```python
from build123d import *

# Parameters (mm, degrees)
CYLINDER005_R          = 1.7
CYLINDER005_DEPTH      = 20
CYLINDER004_R          = 1.7
CYLINDER004_DEPTH      = 36.75
CYLINDER003_R          = 1.7
CYLINDER003_DEPTH      = 39.75
CYLINDER006_R          = 1.7
CYLINDER006_DEPTH      = 20
CYLINDER001_R          = 8
CYLINDER001_DEPTH      = 5
CYLINDER001_ROLL_ANGLE = -90
CYLINDER_R             = 6
CYLINDER_DEPTH         = 30
CYLINDER_ROLL_ANGLE    = -90
CYLINDER002_R          = 8
CYLINDER002_DEPTH      = 12
CYLINDER002_ROLL_ANGLE = -90
BOX_W                  = 50
BOX_H                  = 15.9
BOX_DEPTH              = 13
POCKET_DEPTH           = 121.108539
CHAMFER_SIZE           = 4
FILLET_R               = 1
POCKET001_DEPTH        = 115.108539
CHAMFER001_SIZE        = 1
CHAMFER002_SIZE        = 0.5
FILLET001_R            = 0.25


with BuildPart() as cilindro005:
    # Cylinder005 → Cylinder005 (new body)
    with BuildSketch(Plane(origin=(-12, 7, 11), x_dir=(1, 0, 0), z_dir=(0, 0, 1))):
        Circle(CYLINDER005_R)
    extrude(amount=CYLINDER005_DEPTH)


with BuildPart() as cilindro004:
    # Cylinder004 → Cylinder004 (new body)
    with BuildSketch(Plane(origin=(-12, 7, 0), x_dir=(1, 0, 0), z_dir=(0, 0, 1))):
        Circle(CYLINDER004_R)
    extrude(amount=CYLINDER004_DEPTH)


with BuildPart() as cilindro003:
    # Cylinder003 → Cylinder003 (new body)
    with BuildSketch(Plane(origin=(12, 7, 0), x_dir=(1, 0, 0), z_dir=(0, 0, 1))):
        Circle(CYLINDER003_R)
    extrude(amount=CYLINDER003_DEPTH)


with BuildPart() as tornillos:
    # Cylinder006 → Cylinder006 (new body)
    with BuildSketch(Plane(origin=(12, 7, 11), x_dir=(1, 0, 0), z_dir=(0, 0, 1))):
        Circle(CYLINDER006_R)
    extrude(amount=CYLINDER006_DEPTH)

    # Fusion001: union Cilindro005, Cilindro004, Cilindro003
    add(cilindro005.part)
    add(cilindro004.part)
    add(cilindro003.part)


with BuildPart() as cilindro001:
    # Cylinder001 → Cylinder001 (new body)
    with BuildSketch(Plane.XY):
        Circle(CYLINDER001_R)
    extrude(amount=CYLINDER001_DEPTH)


with BuildPart() as cilindro001_1:
    # Cylinder001 roll: moved
    add(cilindro001.part.rotate(Axis((0, 0, 0), (1, 0, 0)), CYLINDER001_ROLL_ANGLE))


with BuildPart() as cilindro001_2:
    # Cylinder001 placement: moved
    add(cilindro001_1.part.moved(Location((0, -1, 13))))


with BuildPart() as cilindro:
    # Cylinder → Cylinder (new body)
    with BuildSketch(Plane.XY):
        Circle(CYLINDER_R)
    extrude(amount=CYLINDER_DEPTH)


with BuildPart() as cilindro_1:
    # Cylinder roll: moved
    add(cilindro.part.rotate(Axis((0, 0, 0), (1, 0, 0)), CYLINDER_ROLL_ANGLE))


with BuildPart() as cilindro_2:
    # Cylinder placement: moved
    add(cilindro_1.part.moved(Location((0, -5, 13))))


with BuildPart() as cabeza_hot_end:
    # Cylinder002 → Cylinder002 (new body)
    with BuildSketch(Plane.XY):
        Circle(CYLINDER002_R)
    extrude(amount=CYLINDER002_DEPTH)


with BuildPart() as cabeza_hot_end_1:
    # Cylinder002 roll: moved
    add(cabeza_hot_end.part.rotate(Axis((0, 0, 0), (1, 0, 0)), CYLINDER002_ROLL_ANGLE))


with BuildPart() as cabeza_hot_end_2:
    # Cylinder002 placement: moved
    add(cabeza_hot_end_1.part.moved(Location((0, 9.7, 13))))

    # Fusion: union Cilindro001, Cilindro
    add(cilindro001_2.part)
    add(cilindro_2.part)


with BuildPart() as fillet001:
    # Box → Box (new body)
    with BuildSketch(Plane(origin=(-25, 0, 0), x_dir=(1, 0, 0), z_dir=(0, 0, 1))):
        with Locations((25, 7.95)):
            Rectangle(BOX_W, BOX_H)
    extrude(amount=BOX_DEPTH)

    # Cut: cut cabeza_hot_end
    add(cabeza_hot_end_2.part, mode=Mode.SUBTRACT)

    # Cut001: cut tornillos
    add(tornillos.part, mode=Mode.SUBTRACT)

    # Sketch → Pocket (cut, through all)
    with BuildSketch(Plane.XY.offset(13)):
        with BuildLine():
            ThreePointArc((17, 7), (16.5168, 9.144415), (15.160594, 10.874357))
            Line((9, 15.9), (15.160594, 10.874357))
            Line((25, 15.9), (9, 15.9))
            Line((25, 7), (25, 15.9))
            Line((17, 7), (25, 7))
        make_face()
    pocket = extrude(amount=-POCKET_DEPTH, mode=Mode.SUBTRACT)

    # Mirrored: Pocket across Sketch V_Axis
    add(pocket.mirror(Plane(origin=(0, 0, 13), x_dir=(0, 0, 1), z_dir=(1, 0, 0))), mode=Mode.SUBTRACT)

    # Chamfer
    chamfer_edges = [fillet001.edges().sort_by_distance(p)[0] for p in [
        (0, 15.9, 0),
    ]]
    chamfer(chamfer_edges, length=CHAMFER_SIZE)

    # Fillet
    fillet_edges = [fillet001.edges().sort_by_distance(p)[0] for p in [
        (11.451664, 13.9, 2),
        (-11.451664, 13.9, 2),
    ]]
    fillet(fillet_edges, radius=FILLET_R)

    # Sketch002 → Pocket001 (cut, through all)
    with BuildSketch(Plane(origin=(0, 7, 0), x_dir=(-1, 0, 0), z_dir=(0, 1, 0))):
        Polygon((-25, 13), (-17, 0), (-25, 0), align=None)
    pocket001 = extrude(amount=-POCKET001_DEPTH, mode=Mode.SUBTRACT)

    # Mirrored001: Pocket001 across Sketch002 V_Axis
    add(pocket001.mirror(Plane(origin=(0, 7, 0), x_dir=(0, 1, 0), z_dir=(-1, 0, 0))), mode=Mode.SUBTRACT)

    # Chamfer001
    chamfer001_edges = [fillet001.edges().sort_by_distance(p)[0] for p in [
        (0, 0, 0),
    ]]
    chamfer(chamfer001_edges, length=CHAMFER001_SIZE)

    # Chamfer002
    chamfer002_edges = [fillet001.edges().sort_by_distance(p)[0] for p in [
        (10.3, 7, 0),
        (-13.7, 7, 0),
    ]]
    chamfer(chamfer002_edges, length=CHAMFER002_SIZE)

    # Fillet001
    fillet001_edges = [fillet001.edges().sort_by_distance(p)[0] for p in [
        (0, 9.7, 7),
        (0, 4, 7),
    ]]
    fillet(fillet001_edges, radius=FILLET001_R)


solid = fillet001.part
```
Work out the finished part from the listing and answer in its coordinate system (mm). A direction names the side the tool comes from. Coordinates: 2 decimals unless noted, no trailing zeros. Loops run counter-clockwise (first coordinate to the right, second up) from the corner with the lowest first, then second, coordinate; pieces in that order, holes last. Notation, with made-up numbers: (47.25, 15.25) -> (101.25, 15.25) arc R19 cw to (101.25, 36.25) -> close; hole circle Ø7 at (63, -39). An arc over 180 degrees is marked (long way). Answer as CSV lines item,"result".
Q1. The part is cut by section B-B on z = 6. Write down the section's boundary in (x, y), and give its area (3 significant figures).
Findings:
outline,"(-20.69, 0) -> (-3.87, 0) -> (-3.87, 4) -> (3.87, 4) -> (3.87, 0) -> (20.69, 0) -> (20.69, 7) -> (17, 7) arc R5 ccw to (15.16, 10.87) -> (9, 15.9) -> (3.87, 15.9) -> (3.87, 9.7) -> (-3.87, 9.7) -> (-3.87, 15.9) -> (-9, 15.9) -> (-15.16, 10.87) arc R5 ccw to (-17, 7) -> (-20.69, 7) -> close; hole circle Ø3.4 at (-12, 7); hole circle Ø3.4 at (12, 7)"
area,"441 mm²"
Q2. Each of these flat-tipped pins is pushed along its axis until it touches: pin 1 (4 mm diameter, centred on x = -12, y = 7, fed in from -Z); pin 2 (4 mm diameter, centred on y = 4, z = 3, fed in from +X); pin 3 (4 mm diameter, centred on x = -1.5, z = 8.5, fed in from -Y). Where does it stop, or does it pass through?
Findings:
pin 1,"stops at z = 0.2"
pin 2,"stops at x = 20.08"
pin 3,"stops at y = 4"
Q3. A tool of negligible diameter and unlimited length cuts with its end or side. For faces 5 (the face through (-20, 7, 8)), 6 (the face through (0, 2, 5)), 7 (the face through (20, 7, 8)), 8 (the face through (11.484, 13.714, 1.979)), from which of +Z, -Z, +X, -X, +Y, -Y can it reach the whole face along a straight path? Write none if from no direction.
Findings:
face 5,"+Z, -Z, -X, +Y"
face 6,"+Z, -Y"
face 7,"+Z, -Z, +X, +Y"
face 8,"-Z, +X, +Y"
Q4. Find the intervals of material crossed by probe 1 along X at (y, z) = (6, 11.75); probe 2 along Y at (x, z) = (-12, 9.5); probe 3 along X at (y, z) = (1, 8.5), in increasing order.
Findings:
probe 1,"x = -24.23 to -13.37, -10.63 to -5.87, 5.87 to 10.63, 13.37 to 24.23"
probe 2,"y = 0 to 5.3, 8.7 to 13.45"
probe 3,"x = -22.23 to -6.61, 6.61 to 22.23"
Q5. The part is cut by section C-C on z = 10.5. State how many separate pieces and enclosed holes the cut face has, and give its area (3 significant figures).
Findings:
separate pieces,"2"
enclosed holes,"2"
area,"342 mm²"
Q6. The part is cut by section A-A on x = 0. Write down the section's boundary in (y, z), and give its area (3 significant figures).
Findings:
outline,"(0, 1) -> (1, 0) -> (11.9, 0) -> (15.9, 4) -> (15.9, 5) -> (9.7, 5) -> (9.7, 6.75) arc R0.25 ccw to (9.45, 7) -> (4.25, 7) arc R0.25 ccw to (4, 6.75) -> (4, 5) -> (0, 5) -> close"
area,"82.4 mm²"
Q7. For a pull along X with two mould halves and no side action, classify faces 1 (the face through (21.056, 3.549, 6.591)), 2 (the face through (-0.2, 13.9, 2)), 3 (the face through (0, 7, 7)), 4 (the face through (0, 13, 5)) as +X half, -X half, draft (parallel to the pull), parting line (faces both ways), or undercut.
Findings:
face 1,"+X half"
face 2,"draft"
face 3,"undercut"
face 4,"undercut"
